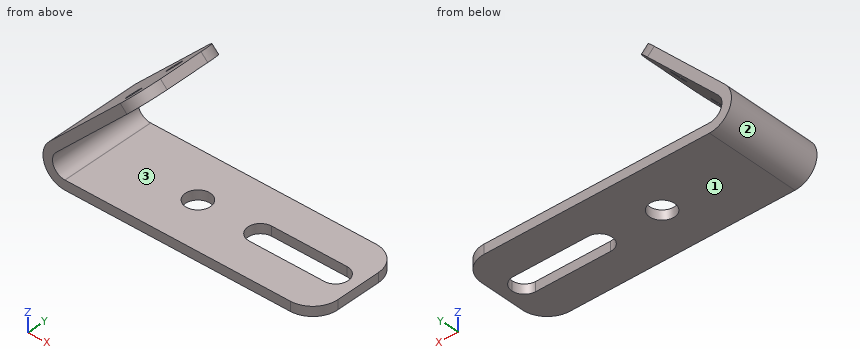
```python
from build123d import *

# Parameters (mm, degrees)
F1_DEPTH = 241.935
F2_R     = 63.5
F3_DEPTH = 48.261
F4_R     = 38.1
F5_DEPTH = 48.26
F6_R     = 127
F7_R     = 127


# Not quite as in the source:
# - a pattern or mirror of a feature is missing from the dataset's text; its kind, count and spacing are read off the source's solid


with BuildPart() as f1:
    # F0 (on Front) → F1 (new body, symmetric)
    with BuildSketch(Plane.XZ):
        with BuildLine():
            Line((-1270, 0), (0, 0))
            Line((0, 0), (0, 48.26))
            Line((0, 48.26), (-1270, 48.26))
            ThreePointArc((-1270, 48.26), (-1328.6663503145, 87.4596020448), (-1314.9012806053, 156.6612806053))
            Line((-1314.9012806053, 156.6612806053), (-865.8884745519, 605.6740866588))
            Line((-865.8884745519, 605.6740866588), (-900.013447812, 639.7990599189))
            Line((-900.013447812, 639.7990599189), (-1349.0262538654, 190.7862538654))
            ThreePointArc((-1349.0262538654, 190.7862538654), (-1373.2527765535, 68.9912995989), (-1270, 0))
        make_face()
    extrude(amount=F1_DEPTH, both=True)

    # F2 (on face) → F3 (cut, through all)
    with BuildSketch(Plane.XY.offset(48.26)):
        with Locations((-812.8, 0)):
            Circle(F2_R)
        with BuildLine():
            ThreePointArc((-495.3, -63.5), (-450.3987193947, -44.9012806053), (-431.8, 0))
            ThreePointArc((-431.8, 0), (-450.3987193947, 44.9012806053), (-495.3, 63.5))
            ThreePointArc((-495.3, 63.5), (-558.8, 0), (-495.3, -63.5))
        make_face()
        with BuildLine():
            ThreePointArc((-495.3, 63.5), (-450.3987193947, 44.9012806053), (-431.8, 0))
            ThreePointArc((-431.8, 0), (-450.3987193947, -44.9012806053), (-495.3, -63.5))
            Line((-495.3, -63.5), (-114.3, -63.5))
            ThreePointArc((-114.3, -63.5), (-177.8, 0), (-114.3, 63.5))
            Line((-114.3, 63.5), (-495.3, 63.5))
        make_face()
        with BuildLine():
            ThreePointArc((-50.8, 0), (-69.3987193947, 44.9012806053), (-114.3, 63.5))
            ThreePointArc((-114.3, 63.5), (-177.8, 0), (-114.3, -63.5))
            ThreePointArc((-114.3, -63.5), (-69.3987193947, -44.9012806053), (-50.8, 0))
        make_face()
    extrude(amount=-F3_DEPTH, mode=Mode.SUBTRACT)

    # F4 (on face) → F5 (cut, through all)
    with BuildSketch(Plane(origin=(-769.9062538654, 0, 769.9062538654), x_dir=(0, -1, 0), z_dir=(-0.7071067812, 0, 0.7071067812))):
        with Locations((114.3, -374.4993582415)):
            Circle(F4_R)
    f5 = extrude(amount=-F5_DEPTH, mode=Mode.SUBTRACT)

    # F5_copies: F5 across plane
    add(f5.mirror(Plane.ZX), mode=Mode.SUBTRACT)

    # F6
    f6_edges = [f1.edges().sort_by_distance(p)[0] for p in [
        (-882.950961, 241.935, 622.736573),
        (-882.950961, -241.935, 622.736573),
    ]]
    fillet(f6_edges, radius=F6_R)

    # F7
    f7_edges = [f1.edges().sort_by_distance(p)[0] for p in [
        (0, 241.935, 24.13),
        (0, -241.935, 24.13),
    ]]
    fillet(f7_edges, radius=F7_R)


solid = f1.part
```
Can you work these out from the model? Positions are in its coordinate system, mm. Face numbers are marked on the shaded views. Round coordinates to 2 decimals unless told otherwise and drop trailing zeros. Order: outer loops, then holes, each group sorted by start corner. A loop starts at its lowest first (then second) coordinate and runs counter-clockwise, first axis right, second up.
(1) We'd pull the mould along Z, two halves only. Please class the marked faces 1, 2 and 3: +Z half, -Z half, draft (parallel to the pull), parting line (faces both ways), or undercut.
Results are:
face 1: -Z half
face 2: parting line
face 3: undercut
(2) If we section it at C-C (y = -39.5): Please give me the cut outline in (x, z).
Results are:
outline: (-1349.03, 190.79) arc R111.76 ccw to (-1270, 0) - (-862.52, 0) - (-862.52, 48.26) - (-1270, 48.26) arc R63.5 cw to (-1314.9, 156.66) - (-865.89, 605.67) - (-900.01, 639.8) - close; (-763.08, 0) - (-545.02, 0) - (-545.02, 48.26) - (-763.08, 48.26) - close; (-64.58, 0) - (0, 0) - (0, 48.26) - (-64.58, 48.26) - close
(3) If we section it at A-A (x = -812.8): Please give me the cut outline in (y, z) (3 decimals), plus the area to 3 significant figures.
Results are:
outline: (-241.935, 0) - (-63.5, 0) - (-63.5, 48.26) - (-241.935, 48.26) - close; (63.5, 0) - (241.935, 0) - (241.935, 48.26) - (63.5, 48.26) - close
area: 17,200 mm2
(4) If we section it at D-D (z = 141): Please give me the cut outline in (x, y) (3 decimals), plus the area to 3 significant figures.
Results are:
outline: (-1377.867, -241.935) - (-1326.367, -241.935) - (-1326.367, 241.935) - (-1377.867, 241.935) - close
area: 24,900 mm2
(5) I'm going to push flat-ended pins straight in: pin 1 (12 mm diameter, centred on y = 189, z = 93, fed in from +X); pin 2 (4 mm diameter, centred on y = 84.5, z = 382.5, fed in from -X); pin 3 (2 mm diameter, centred on y = -152.5, z = 71, fed in from -X). Where does each tip first touch, or does it pass through?
Results are:
pin 1: stops at x = -1328.47
pin 2: stops at x = -1159.31
pin 3: stops at x = -1374.45
(6) If I drill on L1, parallel to Y at x = -812.8, z = 26.5 (3 decimals); L2, parallel to Z at x = -189.5, y = -65; L3, parallel to Z at x = -1323, y = 86 (1 decimal), over which ranges is the centre line in solid material (lowest first)?
Results are:
L1: y = -241.935 to -63.5, 63.5 to 241.935
L2: z = 0 to 48.26
L3: z = 13.4 to 76.8, 146.7 to 216.8
(7) If we section it at B-B (y = 139): Please give me the cut outline in (x, z).
Results are:
outline: (-1349.03, 190.79) arc R111.76 ccw to (-1270, 0) - (-2.3, 0) - (-2.3, 48.26) - (-1270, 48.26) arc R63.5 cw to (-1314.9, 156.66) - (-1021.1, 450.46) - (-1055.23, 484.58) - close; (-1014.2, 525.61) - (-980.08, 491.48) - (-867.52, 604.05) - (-901.64, 638.17) - close
